Design review of the part built by this model. Coordinates are the model's own, in mm. A direction names the side the tool comes from. Round coordinates to 2 decimals unless told otherwise and drop trailing zeros. Order: outer loops, then holes, each group sorted by start corner. A loop starts at its lowest first (then second) coordinate and runs counter-clockwise, first axis right, second up. Notation, with made-up numbers: M 44.5,-7.5 L 95.5,-7.5 A28 cw 95.5,11.5 Z; hole C -25.5,15.5 d5. An arc over 180 degrees is marked long. Write each question's results on one line, items separated by ' | '. Start each with the question number.
Item 1: Take a section at C-C, the plane z = 80.63. Write out the cut boundary in (x, y), plus the area to 3 significant figures.
Item 2: Take a section at A-A, the plane y = -1.1. Write out the cut boundary in (x, z).
Item 3: Take a section at B-B, the plane z = 46.88. Write out the cut boundary in (x, y), plus the area to 3 significant figures.
Item 4: Clearance check with flat-ended pins moving along their axes: pin 1 (0.5 mm diameter, centred on y = -1, z = 13.5, fed in from -X); pin 2 (12 mm diameter, centred on x = 19.5, z = 35, fed in from +Y); pin 3 (0.8 mm diameter, centred on x = 30, y = -1, fed in from -Z); pin 4 (0.8 mm diameter, centred on y = -1, z = 76.5, fed in from +X). State where each tip first meets the part, or that it passes through.
Item 5: Wall thickness on line 1 (Z direction, x = 0, y = -0.35); line 2 (X direction, y = -0.05, z = 18); line 3 (X direction, y = -0.5, z = 46.88): over which ranges is each line inside the solid? List them lowest first. Write a range as [from, to].
Item 6: Machinability: for faces 1 (the flat face through (-30, -1, 81.63)), 2 (the flat face through (30, -1, 23.63)), 3 (the flat face through (-28.75, -1, 12)), 4 (the flat face through (28.75, -1, 76)), which of the approach directions +Z, -Z, +X, -X, +Y, -Y give a long, thin tool a straight path to every point of the face, cutting with its end or side? Answer none if there is none.
Item 7: The part is to be moulded in two halves that separate along Z. For faces 5 (the flat face through (0, -1, 85.43)), 6 (the flat face through (31.55, -1, 47)), 7 (the cylindrical face through (-27.75, -0.79, 71.15)), 8 (the flat face through (-30, -1, 70.13)), say which applies: +Z half, -Z half, draft (parallel to the pull), parting line (faces both ways), or undercut.
```python
from build123d import *

# Parameters (mm, degrees)
PAD009_DEPTH    = 1.6
SKETCH029_R     = 1.6
POCKET014_DEPTH = 1.601


with BuildPart() as part:
    # Sketch028 → Pad009 (new body)
    with BuildSketch(Plane.XZ):
        with BuildLine():
            Line((0, 1.48), (27.75, 1.48))
            Line((27.75, 1.48), (28.75, 2.48))
            Line((28.75, 2.48), (28.75, 21.63))
            ThreePointArc((28.75, 23.63), (27.75, 22.63), (28.75, 21.63))
            Line((28.75, 23.63), (31.55, 23.63))
            Line((31.55, 23.63), (31.55, 70.13))
            Line((31.55, 70.13), (28.75, 70.13))
            ThreePointArc((28.75, 72.13), (27.75, 71.13), (28.75, 70.13))
            Line((28.75, 72.13), (28.75, 79.63))
            ThreePointArc((28.75, 81.63), (27.75, 80.63), (28.75, 79.63))
            Line((28.75, 81.63), (31.55, 81.63))
            Line((31.55, 81.63), (31.55, 85.43))
            Line((31.55, 85.43), (0, 85.43))
            Line((0, 85.43), (0, 1.48))
        make_face()
    pad009 = extrude(amount=PAD009_DEPTH)

    # Mirrored002: Pad009 across Sketch028 V_Axis
    add(pad009.mirror(Plane(origin=(0, 0, 0), x_dir=(0, -1, 0), z_dir=(1, 0, 0))))

    # Sketch029 → Pocket014 (cut, through all)
    with BuildSketch(Plane.XZ):
        with Locations((0, 46.88)):
            Circle(SKETCH029_R)
    extrude(amount=POCKET014_DEPTH, mode=Mode.SUBTRACT)


solid = part.part
```
Results list:
1) outline: M -27.75,-1.6 L 27.75,-1.6 L 27.75,0 L -27.75,0 Z | area: 88.8 mm²
2) outline: M -31.55,23.63 L -28.75,23.63 A1 cw -28.75,21.63 L -28.75,2.48 L -27.75,1.48 L 27.75,1.48 L 28.75,2.48 L 28.75,21.63 A1 cw 28.75,23.63 L 31.55,23.63 L 31.55,70.13 L 28.75,70.13 A1 cw 28.75,72.13 L 28.75,79.63 A1 cw 28.75,81.63 L 31.55,81.63 L 31.55,85.43 L -31.55,85.43 L -31.55,81.63 L -28.75,81.63 A1 cw -28.75,79.63 L -28.75,72.13 A1 cw -28.75,70.13 L -31.55,70.13 Z; hole C 0,46.88 d3.2
3) outline: M -31.55,-1.6 L -1.6,-1.6 L -1.6,0 L -31.55,0 Z; M 1.6,-1.6 L 31.55,-1.6 L 31.55,0 L 1.6,0 Z | area: 95.8 mm²
4) pin 1: x = -28.75 | pin 2: y = 0 | pin 3: z = 23.63 | pin 4: x = 28.75
5) line 1: [1.48, 45.28], [48.48, 85.43] | line 2: [-28.75, 28.75] | line 3: [-31.55, -1.6], [1.6, 31.55]
6) face 1: -X, +Y, -Y | face 2: -Z, +X, +Y, -Y | face 3: -Z, -X, +Y, -Y | face 4: +X, +Y, -Y
7) face 5: +Z half | face 6: draft | face 7: undercut | face 8: undercut
